Geometry: final body of the model. Coordinates: model frame, mm. A direction names the side the tool comes from. Round coordinates to 2 decimals unless told otherwise and drop trailing zeros. Loops run counter-clockwise (first coordinate to the right, second up) from the corner with the lowest first, then second, coordinate; pieces in that order, holes last. Notation, with made-up numbers: (-16, -21) - (27, -21) arc R28 ccw to (27, 2) - close; hole circle Ø4 at (8.5, 44). An arc over 180 degrees is marked (long way). Answer in a Markdown table with one row per item. Add a question column.
from build123d import *

# Parameters (mm, degrees)
SKETCH1_W           = 25.4
SKETCH1_H           = 4.572
BOSS_EXTRUDE1_DEPTH = 76.2
BOSS_EXTRUDE3_DEPTH = 4.572
FILLET3_R           = 6.35
SKETCH5_R           = 2.54
CUT_EXTRUDE2_DEPTH  = 112.853479088


with BuildPart() as part:
    # Sketch1 → Boss-Extrude1 (new body)
    with BuildSketch(Plane.XY):
        with Locations((12.7, 2.286)):
            Rectangle(SKETCH1_W, SKETCH1_H)
    extrude(amount=BOSS_EXTRUDE1_DEPTH)

    # Sketch4 → Boss-Extrude3 (add)
    with BuildSketch(Plane(origin=(25.4, 0, 0), x_dir=(0, 0, -1), z_dir=(1, 0, 0))):
        Polygon((-76.2, 0), (-76.2, 4.572), (-12.7, 76.2), (0, 76.2), (0, 0), align=None)
    extrude(amount=BOSS_EXTRUDE3_DEPTH)

    # Fillet3
    fillet3_edges = [part.edges().sort_by_distance(p)[0] for p in [
        (27.686, 76.2, 0),
        (27.686, 76.2, 12.7),
    ]]
    fillet(fillet3_edges, radius=FILLET3_R)

    # Sketch5 → Cut-Extrude2 (cut, through all)
    with BuildSketch(Plane(origin=(29.972, 0, 0), x_dir=(0, 0, -1), z_dir=(1, 0, 0))):
        with Locations((-8.255, 69.85)):
            Circle(SKETCH5_R)
    extrude(amount=-CUT_EXTRUDE2_DEPTH, mode=Mode.SUBTRACT)


solid = part.part
1) Section A-A, the plane x = 27. Return the cut outline in (y, z) (3 decimals).
2) Section C-C, the plane x = 15.5. Return the cut outline in (y, z).
3) Material intervals for line 1 along Y through (x, z) = (6.5, 58); line 2 along X through (y, z) = (60, 15); line 3 along Y through (x, z) = (25.75, 15.5), sorted ascending. Write a range as from..to.
4) Section D-D, the plane y = 59. Return the cut outline in (x, z), and give its area (3 significant figures).
5) Reachability of faces 1 (the flat face through (25.4, 33, 29)), 2 (the flat face through (0, 2, 38)) from +Z, -Z, +X, -X, +Y, -Y: full face, straight path, thin tool, end or side. Return the list, or none.
6) Contact query for flat-ended pins moving along their axis: pin 1 Ø1.5 at (y, z) = (23, 34) entering from -X; pin 2 Ø6 at (x, z) = (9.5, 49.5) entering from +Y. Output: stop coordinate, or through.
7) Section B-B, the plane z = 59. Return the cut outline in (x, y), and give its area (3 significant figures).
Evaluation:
| question | item | result |
|---|---|---|
| 1 | outline | (0, 0) - (69.85, 0) arc R6.35 ccw to (76.2, 6.35) - (76.2, 9.843) arc R6.35 ccw to (74.062, 14.595) - (4.572, 76.2) - (0, 76.2) - close; hole circle Ø5.08 at (69.85, 8.255) |
| 2 | outline | (0, 0) - (4.57, 0) - (4.57, 76.2) - (0, 76.2) - close |
| 3 | line 1 | y = 0..4.57 |
| 3 | line 2 | x = 25.4..29.97 |
| 3 | line 3 | y = 0..73.04 |
| 4 | outline | (25.4, 0) - (29.97, 0) - (29.97, 27.95) - (25.4, 27.95) - close |
| 4 | area | 128 mm² |
| 5 | face 1 | +Z, -Z, -X, +Y |
| 5 | face 2 | +Z, -Z, -X, +Y, -Y |
| 6 | pin 1 | stops at x = 25.4 |
| 6 | pin 2 | stops at y = 4.57 |
| 7 | outline | (0, 0) - (29.97, 0) - (29.97, 23.97) - (25.4, 23.97) - (25.4, 4.57) - (0, 4.57) - close |
| 7 | area | 226 mm² |
